from build123d import *

# Parameters (mm, degrees)
CUT_EXTRUDE1_REACH = 11.621
CHAMFER1_SIZE      = 0.225
FILLET1_R          = 0.65


with BuildPart() as part:
    # Boss-Extrude1: read off the stored shape, not the designer's step
    # Boss-Extrude1 outline → Boss-Extrude1 (revolve)
    with BuildSketch(Plane.XY):
        with BuildLine():
            ThreePointArc((2.378097174, 1.12), (1.213027841, 1.478802074), (0, 1.6))
            Line((0, 1.6), (0, -8))
            Line((0, -8), (1.3, -8))
            Line((1.3, -8), (1.3, 0))
            Line((1.3, 0), (2.378097174, 0))
            ThreePointArc((2.378097174, 0), (2.75, 0.56), (2.378097174, 1.12))
        make_face()
    revolve(axis=Axis((0, 0, 0), (0, 1, 0)))

    # Sketch2 → Cut-Extrude1 (cut, up to next)
    with BuildSketch(Plane.XZ.offset(-0.8), mode=Mode.PRIVATE) as cut_extrude1_sk1:
        with BuildLine():
            Line((-0.269238816, 1.526437179), (-0.269238816, 0.269238816))
            Line((-0.269238816, 0.269238816), (-1.526437179, 0.269238816))
            ThreePointArc((-1.526437179, 0.269238816), (-1.55, 0), (-1.526437179, -0.269238816))
            Line((-1.526437179, -0.269238816), (-0.269238816, -0.269238816))
            Line((-0.269238816, -0.269238816), (-0.269238816, -1.526437179))
            ThreePointArc((-0.269238816, -1.526437179), (0, -1.55), (0.269238816, -1.526437179))
            Line((0.269238816, -1.526437179), (0.269238816, -0.269238816))
            Line((0.269238816, -0.269238816), (1.526437179, -0.269238816))
            ThreePointArc((1.526437179, -0.269238816), (1.55, 0), (1.526437179, 0.269238816))
            Line((1.526437179, 0.269238816), (0.269238816, 0.269238816))
            Line((0.269238816, 0.269238816), (0.269238816, 1.526437179))
            ThreePointArc((0.269238816, 1.526437179), (0, 1.55), (-0.269238816, 1.526437179))
        make_face()
    cut_extrude1_tool1 = extrude(cut_extrude1_sk1.sketch, amount=-CUT_EXTRUDE1_REACH, mode=Mode.PRIVATE) & part.part
    add(cut_extrude1_tool1.solids().sort_by_distance((0, 0.8, 0))[0], mode=Mode.SUBTRACT)

    # Chamfer1
    chamfer1_edges = [part.edges().sort_by_distance(p)[0] for p in [
        (-1.3, -8, 0),
    ]]
    chamfer(chamfer1_edges, length=CHAMFER1_SIZE)

    # Fillet1
    fillet1_edges = [part.edges().sort_by_distance(p)[0] for p in [
        (-0.269238816, 1.194082552, 0.269238816),
        (0.269238816, 1.194082552, 0.269238816),
        (-0.269238816, 1.194082552, -0.269238816),
        (0.269238816, 1.194082552, -0.269238816),
    ]]
    fillet(fillet1_edges, radius=FILLET1_R)


solid = part.part
Read the model definition and answer for the solid it produces. Units are mm, in the model's axes. Give positions to 0.01 mm unless a question says otherwise; leave off trailing zeros. Write each loop counter-clockwise with the first axis right and the second up, starting at its lowest first coordinate (ties: lowest second). Pieces come first, ordered by that corner, then holes. Notation, with made-up numbers: (-2, -13.5) - (34, -13.5) arc R28 ccw to (34, 25.5) - close; hole circle Ø10 at (-29.5, -6). An arc over 180 degrees is marked (long way). Return JSON: item names as keys, results as strings.
Q1. A cutting plane is placed at A-A, the plane z = 0. Determine the outline of the cut face in (x, y) (3 decimals), and give its area (3 significant figures).
Reply:
{"outline": "(-2.378, 0) - (-1.3, 0) - (-1.3, -7.775) - (-1.075, -8) - (1.075, -8) - (1.3, -7.775) - (1.3, 0) - (2.378, 0) arc R0.608 ccw to (2.378, 1.12) arc R6.131 ccw to (1.55, 1.401) - (1.55, 0.8) - (-1.55, 0.8) - (-1.55, 1.401) arc R6.131 ccw to (-2.378, 1.12) arc R0.608 ccw to start", "area": "25.9 mm²"}
Q2. For a pull along X with two mould halves and no side action, classify faces 1 (the face through (-2, 0, 0)), 2 (the face through (0, 0.8, 0)), 3 (the face through (-0.17, -3.83, -1.29)) as released by +X, released by -X, zero draft, split by the parting line, or undercut.
Reply:
{"face 1": "zero draft", "face 2": "undercut", "face 3": "split by the parting line"}
Q3. A cutting plane is placed at B-B, the plane x = 0. Determine the outline of the cut face in (y, z) (3 decimals), and give its area (3 significant figures).
Reply:
{"outline": "(-8, -1.075) - (-7.775, -1.3) - (0, -1.3) - (0, -2.378) arc R0.608 ccw to (1.12, -2.378) arc R6.131 ccw to (1.401, -1.55) - (0.8, -1.55) - (0.8, 1.55) - (1.401, 1.55) arc R6.131 ccw to (1.12, 2.378) arc R0.608 ccw to (0, 2.378) - (0, 1.3) - (-7.775, 1.3) - (-8, 1.075) - close", "area": "25.9 mm²"}
Q4. Given P1, Ø3, axis at x = -1, y = -3, coming from the -Z side; P2, Ø1.6, axis at x = 0.5, z = -0.5, coming from the +Y side; P3, Ø0.5, axis at y = 1, z = 1.5, coming from the +X side; P4, Ø0.5, axis at x = -1.5, y = 1, coming from the +Z side, each flat-ended and moving along its own axis, determine where each tip first touches the part or whether it passes through.
Reply:
{"P1": "z = -1.3", "P2": "y = 1.57", "P3": "x = 2.34", "P4": "z = 2.34"}
Q5. Consider line 1 along Z through (x, y) = (-0.05, -7); line 2 along Y through (x, z) = (-0.8, 0.25). Determine where each line is inside the solid, lowest interval first. Write a range as [from, to].
Reply:
{"line 1": "[-1.3, 1.3]", "line 2": "[-8, 0.8]"}
Q6. A cutting plane is placed at C-C, the plane y = -5.25. Determine the outline of the cut face in (x, z), and give its area (3 significant figures).
Reply:
{"outline": "circle Ø2.6 at (0, 0)", "area": "5.31 mm²"}
